from build123d import *

# Parameters (mm, degrees)
SKETCH_2_W                       = 240
SKETCH_2_H                       = 105
EXTRUDE_1_DEPTH                  = 6
SKETCH_22_R                      = 4.1
CUT_EXTRUDE_3_DEPTH              = 223.650914893
PATTERN_LINEAR_2_COUNT           = 5
PATTERN_LINEAR_2_PITCH           = 55
PATTERN_LINEAR_3_COPY_1_SKETCH_R = 4.1
PATTERN_LINEAR_3_COPY_1_DEPTH    = 223.650914893
PATTERN_LINEAR_3_COPY_2_SKETCH_R = 4.1
PATTERN_LINEAR_3_COPY_2_DEPTH    = 223.650914893
PATTERN_LINEAR_3_COPY_3_SKETCH_R = 4.1
PATTERN_LINEAR_3_COPY_3_DEPTH    = 223.650914893
PATTERN_LINEAR_3_COPY_4_SKETCH_R = 4.1
PATTERN_LINEAR_3_COPY_4_DEPTH    = 223.650914893
PATTERN_LINEAR_3_COPY_5_SKETCH_R = 4.1
PATTERN_LINEAR_3_COPY_5_DEPTH    = 223.650914893
PATTERN_LINEAR_3_COPY_6_SKETCH_R = 4.1
PATTERN_LINEAR_3_COPY_6_DEPTH    = 223.650914893
PATTERN_LINEAR_3_COPY_7_SKETCH_R = 4.1
PATTERN_LINEAR_3_COPY_7_DEPTH    = 223.650914893
PATTERN_LINEAR_3_COPY_8_SKETCH_R = 4.1
PATTERN_LINEAR_3_COPY_8_DEPTH    = 223.650914893
SKETCH_18_R                      = 6.5
EXTRUDE_5_DEPTH                  = 45.6
SKETCH_25_W                      = 110
SKETCH_25_H                      = 8.2
CUT_EXTRUDE_4_DEPTH              = 229.473171078
MIRROR_27_COPY_1_SKETCH_W        = 110
MIRROR_27_COPY_1_SKETCH_H        = 8.2
MIRROR_27_COPY_1_DEPTH           = 229.473171078
MIRROR_27_COPY_2_SKETCH_W        = 110
MIRROR_27_COPY_2_SKETCH_H        = 8.2
MIRROR_27_COPY_2_DEPTH           = 229.473171078


with BuildPart() as part:
    # 草图2 → 凸台-拉伸1 (new body)
    with BuildSketch(Plane(origin=(0, 0, 0), x_dir=(1, 0, 0), z_dir=(0, 1, 0))):
        with Locations((-85.476378725, 33.038808084)):
            Rectangle(SKETCH_2_W, SKETCH_2_H)
    extrude(amount=EXTRUDE_1_DEPTH)

    # 草图22 → 切除-拉伸3 (cut, through all)
    with BuildSketch(Plane(origin=(0, 0, 0), x_dir=(1, 0, 0), z_dir=(0, 1, 0))):
        with Locations(Location((-195.476378725, 78.038808084, 0), (0, 0, 270))):
            Circle(SKETCH_22_R)
    cut_extrude_3 = extrude(amount=CUT_EXTRUDE_3_DEPTH, mode=Mode.SUBTRACT)

    # 镜向18: 切除-拉伸3 across plane
    add(cut_extrude_3.mirror(Plane.XY.offset(-33.038808084)), mode=Mode.SUBTRACT)

    # 阵列(线性)2: 切除-拉伸3 ×5
    with Locations(*[(i * PATTERN_LINEAR_2_PITCH, 0, 0) for i in range(1, PATTERN_LINEAR_2_COUNT)]):
        add(cut_extrude_3, mode=Mode.SUBTRACT)

    # 阵列(线性)3 copy 1 sketch → 阵列(线性)3 copy 1 (cut, through all)
    with BuildSketch(Plane(origin=(55, 0, -66.077616169), x_dir=(1, 0, 0), z_dir=(0, 1, 0))):
        with Locations((-195.476378725, -78.038808084)):
            Circle(PATTERN_LINEAR_3_COPY_1_SKETCH_R)
    extrude(amount=PATTERN_LINEAR_3_COPY_1_DEPTH, mode=Mode.SUBTRACT)

    # 阵列(线性)3 copy 2 sketch → 阵列(线性)3 copy 2 (cut, through all)
    with BuildSketch(Plane(origin=(110, 0, -66.077616169), x_dir=(1, 0, 0), z_dir=(0, 1, 0))):
        with Locations((-195.476378725, -78.038808084)):
            Circle(PATTERN_LINEAR_3_COPY_2_SKETCH_R)
    extrude(amount=PATTERN_LINEAR_3_COPY_2_DEPTH, mode=Mode.SUBTRACT)

    # 阵列(线性)3 copy 3 sketch → 阵列(线性)3 copy 3 (cut, through all)
    with BuildSketch(Plane(origin=(165, 0, -66.077616169), x_dir=(1, 0, 0), z_dir=(0, 1, 0))):
        with Locations((-195.476378725, -78.038808084)):
            Circle(PATTERN_LINEAR_3_COPY_3_SKETCH_R)
    extrude(amount=PATTERN_LINEAR_3_COPY_3_DEPTH, mode=Mode.SUBTRACT)

    # 阵列(线性)3 copy 4 sketch → 阵列(线性)3 copy 4 (cut, through all)
    with BuildSketch(Plane(origin=(220, 0, -66.077616169), x_dir=(1, 0, 0), z_dir=(0, 1, 0))):
        with Locations((-195.476378725, -78.038808084)):
            Circle(PATTERN_LINEAR_3_COPY_4_SKETCH_R)
    extrude(amount=PATTERN_LINEAR_3_COPY_4_DEPTH, mode=Mode.SUBTRACT)

    # 阵列(线性)3 copy 5 sketch → 阵列(线性)3 copy 5 (cut, through all)
    with BuildSketch(Plane(origin=(55, 0, 0), x_dir=(1, 0, 0), z_dir=(0, 1, 0))):
        with Locations(Location((-195.476378725, 78.038808084, 0), (0, 0, 270))):
            Circle(PATTERN_LINEAR_3_COPY_5_SKETCH_R)
    extrude(amount=PATTERN_LINEAR_3_COPY_5_DEPTH, mode=Mode.SUBTRACT)

    # 阵列(线性)3 copy 6 sketch → 阵列(线性)3 copy 6 (cut, through all)
    with BuildSketch(Plane(origin=(110, 0, 0), x_dir=(1, 0, 0), z_dir=(0, 1, 0))):
        with Locations(Location((-195.476378725, 78.038808084, 0), (0, 0, 270))):
            Circle(PATTERN_LINEAR_3_COPY_6_SKETCH_R)
    extrude(amount=PATTERN_LINEAR_3_COPY_6_DEPTH, mode=Mode.SUBTRACT)

    # 阵列(线性)3 copy 7 sketch → 阵列(线性)3 copy 7 (cut, through all)
    with BuildSketch(Plane(origin=(165, 0, 0), x_dir=(1, 0, 0), z_dir=(0, 1, 0))):
        with Locations(Location((-195.476378725, 78.038808084, 0), (0, 0, 270))):
            Circle(PATTERN_LINEAR_3_COPY_7_SKETCH_R)
    extrude(amount=PATTERN_LINEAR_3_COPY_7_DEPTH, mode=Mode.SUBTRACT)

    # 阵列(线性)3 copy 8 sketch → 阵列(线性)3 copy 8 (cut, through all)
    with BuildSketch(Plane(origin=(220, 0, 0), x_dir=(1, 0, 0), z_dir=(0, 1, 0))):
        with Locations(Location((-195.476378725, 78.038808084, 0), (0, 0, 270))):
            Circle(PATTERN_LINEAR_3_COPY_8_SKETCH_R)
    extrude(amount=PATTERN_LINEAR_3_COPY_8_DEPTH, mode=Mode.SUBTRACT)

    # 草图18 → 凸台-拉伸5 (add)
    with BuildSketch(Plane(origin=(0, 6, 0), x_dir=(1, 0, 0), z_dir=(0, 1, 0))):
        with Locations(Location((-85.476378725, 33.038808084, 0), (0, 0, 270))):
            Circle(SKETCH_18_R)
    extrude(amount=EXTRUDE_5_DEPTH)

    # 草图25 → 切除-拉伸4 (cut, through all)
    with BuildSketch(Plane(origin=(0, 0, 0), x_dir=(1, 0, 0), z_dir=(0, 1, 0))):
        with Locations((-140.476378725, 78.038808084)):
            Rectangle(SKETCH_25_W, SKETCH_25_H)
    cut_extrude_4 = extrude(amount=CUT_EXTRUDE_4_DEPTH, mode=Mode.SUBTRACT)

    # 镜向25: 切除-拉伸4 across plane
    add(cut_extrude_4.mirror(Plane.XY.offset(-33.038808084)), mode=Mode.SUBTRACT)

    # 镜向26: 切除-拉伸4 across plane
    add(cut_extrude_4.mirror(Plane(origin=(-85.476378725, 0, 0), x_dir=(0, 0, 1), z_dir=(1, 0, 0))), mode=Mode.SUBTRACT)

    # 镜向27 copy 1 sketch → 镜向27 copy 1 (cut, through all)
    with BuildSketch(Plane(origin=(-170.95275745, 0, -66.077616169), x_dir=(-1, 0, 0), z_dir=(0, 1, 0))):
        with Locations((-140.476378725, 78.038808084)):
            Rectangle(MIRROR_27_COPY_1_SKETCH_W, MIRROR_27_COPY_1_SKETCH_H)
    extrude(amount=MIRROR_27_COPY_1_DEPTH, mode=Mode.SUBTRACT)

    # 镜向27 copy 2 sketch → 镜向27 copy 2 (cut, through all)
    with BuildSketch(Plane(origin=(-170.95275745, 0, 0), x_dir=(-1, 0, 0), z_dir=(0, 1, 0))):
        with Locations((-140.476378725, -78.038808084)):
            Rectangle(MIRROR_27_COPY_2_SKETCH_W, MIRROR_27_COPY_2_SKETCH_H)
    extrude(amount=MIRROR_27_COPY_2_DEPTH, mode=Mode.SUBTRACT)


solid = part.part
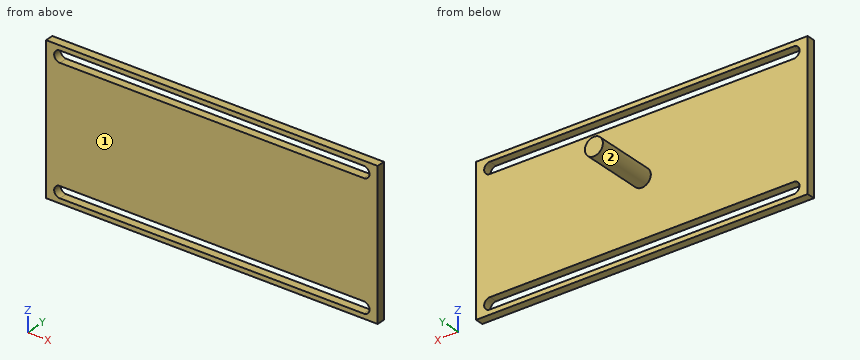
Here's how the part is built. I have some questions about the finished solid (model axes, mm). Face numbers are marked on the shaded views. A direction names the side the tool comes from. Coordinates: 2 decimals unless noted, no trailing zeros. Order: outer loops, then holes, each group sorted by start corner. A loop starts at its lowest first (then second) coordinate and runs counter-clockwise, first axis right, second up.
Item 1: If we section it at B-B on z = -31: List the corners of the cut face in (x, y) for me, plus the area to 3 significant figures.
Result sheet:
outline: (-205.48, 0) - (34.52, 0) - (34.52, 6) - (-79.3, 6) - (-79.3, 51.6) - (-91.65, 51.6) - (-91.65, 6) - (-205.48, 6) - close
area: 2,000 mm2
Item 2: For the marked faces 1 and 2, which set-ups out of +Z, -Z, +X, -X, +Y, -Y let a thin tool reach every point of the face, with its end or its side?
Result sheet:
face 1: +Z, -Z, +X, -X, -Y
face 2: +Y
Item 3: If we section it at C-C on y = 45: List the corners of the cut face in (x, z) for me, plus the area to 3 significant figures.
Result sheet:
outline: circle Ø13 at (-85.48, -33.04)
area: 133 mm2
Item 4: If we section it at D-D on z = -55: List the corners of the cut face in (x, y) for me, plus the area to 3 significant figures.
Result sheet:
outline: (-205.48, 0) - (34.52, 0) - (34.52, 6) - (-205.48, 6) - close
area: 1,440 mm2
Item 5: For P1, Ø12, axis at y = 11, z = -1, coming from the +X side; P2, Ø5, axis at x = 10, z = -32.5, coming from the +Y side, each with a flat end and sliding along its axis, tell me the tip position at first contact or that it passes through.
Result sheet:
P1: stops at x = 34.52
P2: stops at y = 6
Item 6: If we section it at A-A on x = -138: List the corners of the cut face in (y, z) for me.
Result sheet:
outline: (0, -85.54) - (6, -85.54) - (6, -82.14) - (0, -82.14) - close; (0, -73.94) - (6, -73.94) - (6, 7.86) - (0, 7.86) - close; (0, 16.06) - (6, 16.06) - (6, 19.46) - (0, 19.46) - close
Item 7: I need wall thicknesses on line 1 (Z direction, x = 6, y = 3.5); line 2 (Y direction, x = -58.5, z = -15); line 3 (X direction, y = 39, z = -33.5). Which ranges of each line are inside material? Lowest first, please.
Result sheet:
line 1: z = -85.54 to -82.14, -73.94 to 7.86, 16.06 to 19.46
line 2: y = 0 to 6
line 3: x = -91.96 to -78.99
